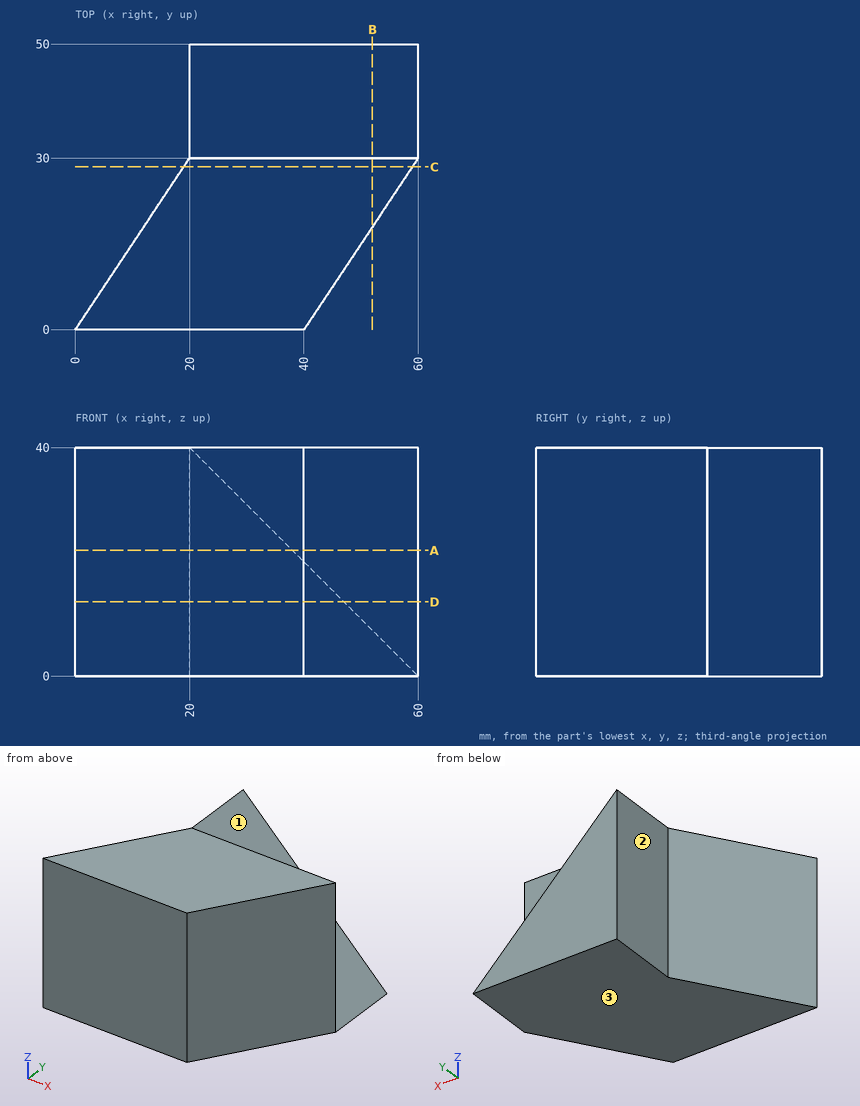
Can you work these out from the drawing? Everything is in mm from the part's minimum corner. A direction names the side the tool comes from. Give positions to 0.01 mm unless a question says otherwise; leave off trailing zeros. Loops run counter-clockwise (first coordinate to the right, second up) from the corner with the lowest first, then second, coordinate; pieces in that order, holes last. Notation, with made-up numbers: (52.25, -22) -> (92.25, -22) arc R27 cw to (92.25, 17) -> close; hole circle Ø4 at (81, 70.5). An arc over 180 degrees is marked (long way). Write item = value, one per line.
1) For the marked faces 1, 2 and 3, which set-ups out of +Z, -Z, +X, -X, +Y, -Y let a thin tool reach every point of the face, with its end or its side?
Check result:
face_1 = +Z, +X, +Y
face_2 = +Z, -Z, -X, +Y
face_3 = -Z, +X, -X, +Y, -Y
2) Suppose I cut it at D-D on z = 13. Write out the boundary of the cut face in (x, y).
Check result:
outline = (0, 0) -> (40, 0) -> (60, 30) -> (47, 30) -> (47, 50) -> (20, 50) -> (20, 30) -> close
3) Will these pins go through, and if not, where does the flat tip stop? pin 1 (6 mm diameter, centred on x = 18, y = 42, fed in from -Z); pin 2 (1.5 mm diameter, centred on y = 42, z = 10.5, fed in from +X); pin 3 (2 mm diameter, centred on x = 29, y = 31.5, fed in from +Z); pin 4 (2 mm diameter, centred on y = 33, z = 24, fed in from +X).
Check result:
pin_1 = 0
pin_2 = 50.25
pin_3 = 32
pin_4 = 37
4) Suppose I cut it at A-A on z = 22. Write out the boundary of the cut face in (x, y), then the cut area to 3 significant figures.
Check result:
outline = (0, 0) -> (40, 0) -> (60, 30) -> (38, 30) -> (38, 50) -> (20, 50) -> (20, 30) -> close
area = 1,560 mm2
5) I need wall thicknesses on L1, parallel to X at y = 20.5, z = 22.5; L2, parallel to X at y = 45, z = 11.5; L3, parallel to Z at x = 24.5, y = 44. Which ranges of each line are inside material? Lowest first, please. Write a range as from..to.
Check result:
L1 = 13.67..53.67
L2 = 20..48.5
L3 = 0..35.5
6) Suppose I cut it at C-C on y = 28.5. Write out the boundary of the cut face in (x, z), then the cut area to 3 significant figures.
Check result:
outline = (19, 0) -> (59, 0) -> (59, 40) -> (19, 40) -> close
area = 1,600 mm2
7) Suppose I cut it at B-B on x = 52. Write out the boundary of the cut face in (y, z), then the cut area to 3 significant figures.
Check result:
outline = (18, 0) -> (50, 0) -> (50, 8) -> (30, 8) -> (30, 40) -> (18, 40) -> close
area = 640 mm2
